Source: CAD feature listing. Evaluate the final solid. Frame: model axes, mm. Give positions to 0.01 mm unless a question says otherwise; leave off trailing zeros. Write each loop counter-clockwise with the first axis right and the second up, starting at its lowest first coordinate (ties: lowest second). Pieces come first, ordered by that corner, then holes. Notation, with made-up numbers: (21.5, 40) -> (47.5, 40) arc R22 ccw to (47.5, 54) -> close; hole circle Ø11 at (74.5, 4). An arc over 180 degrees is marked (long way). Use one line per item in the form item = value. Start each with the question number.
(1) Material intervals for line 1 along X through (y, z) = (2.25, 26.4); line 2 along Z through (x, y) = (19.5, 1.85); line 3 along X through (y, z) = (1.5, 14.5), sorted ascending. Write a range as from..to.
(2) First-contact query: P1, Ø3.5, axis at x = -40, z = 26.4, coming from the +Y side; P2, Ø2.5, axis at x = 20, z = -15, coming from the -Y side. Flat tips, straight axial feed; report the tip coordinate or a pass-through.
(3) Cut plane A-A, the plane x = -20. Output: boundary loops of the cut face in (y, z).
(4) Cut plane B-B, the plane z = -26.4. Output: boundary loops of the cut face in (x, y).
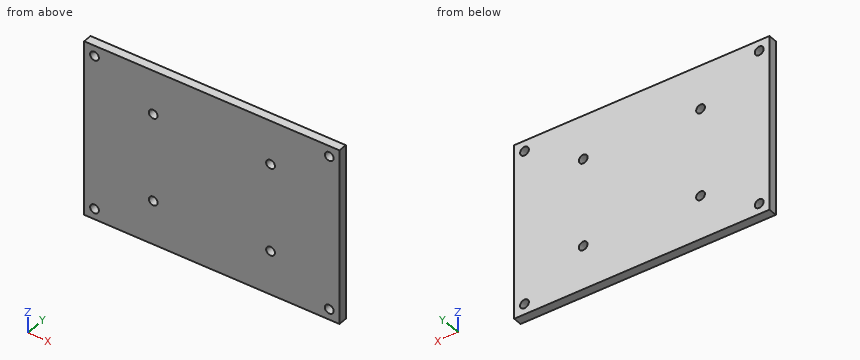
from build123d import *

# Parameters (mm, degrees)
SKETCH_1_W          = 87
SKETCH_1_H          = 60
EXTRUDE_1_DEPTH     = 3
SKETCH_2_R          = 1.5
CUT_EXTRUDE_1_DEPTH = 53.926836293
SKETCH_3_R          = 1.5
CUT_EXTRUDE_2_DEPTH = 53.926836293


with BuildPart() as part:
    # 草图1 → 凸台-拉伸1 (new body)
    with BuildSketch(Plane(origin=(0, 0, 0), x_dir=(1, 0, 0), z_dir=(0, 1, 0))):
        Rectangle(SKETCH_1_W, SKETCH_1_H)
    extrude(amount=EXTRUDE_1_DEPTH)

    # 草图2 → 切除-拉伸1 (cut, through all)
    with BuildSketch(Plane(origin=(0, 3, 0), x_dir=(1, 0, 0), z_dir=(0, 1, 0))):
        with Locations(Location((-40, 26.4, 0), (0, 0, 270))):
            Circle(SKETCH_2_R)
        with Locations(Location((40, 26.4, 0), (0, 0, 270))):
            Circle(SKETCH_2_R)
        with Locations(Location((40, -26.4, 0), (0, 0, 270))):
            Circle(SKETCH_2_R)
        with Locations(Location((-40, -26.4, 0), (0, 0, 270))):
            Circle(SKETCH_2_R)
    extrude(amount=-CUT_EXTRUDE_1_DEPTH, mode=Mode.SUBTRACT)

    # 草图3 → 切除-拉伸2 (cut, through all)
    with BuildSketch(Plane(origin=(0, 3, 0), x_dir=(1, 0, 0), z_dir=(0, 1, 0))):
        with Locations(Location((20, 15, 0), (0, 0, 270))):
            Circle(SKETCH_3_R)
        with Locations(Location((20, -15, 0), (0, 0, 270))):
            Circle(SKETCH_3_R)
        with Locations(Location((-20, 15, 0), (0, 0, 270))):
            Circle(SKETCH_3_R)
        with Locations(Location((-20, -15, 0), (0, 0, 270))):
            Circle(SKETCH_3_R)
    extrude(amount=-CUT_EXTRUDE_2_DEPTH, mode=Mode.SUBTRACT)


solid = part.part
Geometry says:
q1.line_1 = -43.5..-41.5, -38.5..38.5, 41.5..43.5
q1.line_2 = -30..-16.41, -13.59..13.59, 16.41..30
q1.line_3 = -43.5..-21.41, -18.59..18.59, 21.41..43.5
q2.P1 = 3
q2.P2 = through
q3.outline = (0, -30) -> (3, -30) -> (3, -16.5) -> (0, -16.5) -> close; (0, -13.5) -> (3, -13.5) -> (3, 13.5) -> (0, 13.5) -> close; (0, 16.5) -> (3, 16.5) -> (3, 30) -> (0, 30) -> close
q4.outline = (-43.5, 0) -> (-41.5, 0) -> (-41.5, 3) -> (-43.5, 3) -> close; (-38.5, 0) -> (38.5, 0) -> (38.5, 3) -> (-38.5, 3) -> close; (41.5, 0) -> (43.5, 0) -> (43.5, 3) -> (41.5, 3) -> close
